Part model, mm, in its own coordinate system. Face numbers are marked on the shaded views. Round coordinates to 2 decimals unless told otherwise and drop trailing zeros. Loops run counter-clockwise (first coordinate to the right, second up) from the corner with the lowest first, then second, coordinate; pieces in that order, holes last. Notation, with made-up numbers: (6.5, -22.75) -> (30.5, -22.75) arc R33 ccw to (30.5, 12.25) -> close; hole circle Ø4 at (1.5, 48). An arc over 180 degrees is marked (long way). Use a Markdown table: item, result. Add a question column.
Item 1: Two-plate mould, pull along Y, no slides. Class the marked faces 1 and 2: pulls with the +Y half, pulls with the -Y half, needs draft (parallel to the pull), parting line crosses it, or undercut.
Item 2: Cut at C-C, the plane z = -21. List the corners of the cut face in (x, y), plus the area to 3 significant figures.
Item 3: Cut at D-D, the plane y = -20. List the corners of the cut face in (x, z).
Item 4: Flat gauge pins, fed straight in: pin 1 (1 mm diameter, centred on x = 1.5, z = -19, fed in from -Y); pin 2 (15 mm diameter, centred on y = 1, z = 5, fed in from -X); pin 3 (1 mm diameter, centred on x = 4, z = 22.5, fed in from +Y); pin 4 (4 mm diameter, centred on y = 0, z = 20, fed in from -X). Where does each tip first touch, or does it go through?
Item 5: Cut at A-A, the plane z = 0. List the corners of the cut face in (x, y).
Item 6: Probe line 1 (Y direction, x = 3.85, z = 0); line 2 (Z direction, x = 4.8, y = -20); line 3 (Y direction, x = 1.4, z = 21). List the from-to ranges inside material, lowest first. Write a range as [from, to].
```python
from build123d import *

# Parameters (mm, degrees)
SKETCH_2_R               = 2.5
CUT_EXTRUDE_1_DEPTH      = 33.3
PATTERN_CIRCULAR_1_COUNT = 4


with BuildPart() as part:
    # Эскиз1 → Повернуть1 (revolve)
    with BuildSketch(Plane.XY, mode=Mode.PRIVATE) as revolve_1_sk:
        Polygon((6, 0), (6, 35), (3, 35), (3, 32), (0, 32), (0, 15), (2, 15), (2, 0), align=None)
    revolve(revolve_1_sk.sketch.rotate(Axis((0, 0, 0), (1, 0, 0)), 90), axis=Axis((0, 0, 0), (1, 0, 0)))

    # Эскиз2 → Вырез-Вытянуть1 (cut)
    with BuildSketch(Plane.ZY):
        with Locations((0, 20)):
            Circle(SKETCH_2_R)
    cut_extrude_1 = extrude(amount=-CUT_EXTRUDE_1_DEPTH, mode=Mode.SUBTRACT)

    # Круговой массив1: Вырез-Вытянуть1 ×4 about axis
    pattern_circular_1_axis = Axis((0, 0, 0), (1, 0, 0))
    for i in range(1, PATTERN_CIRCULAR_1_COUNT):
        add(cut_extrude_1.rotate(pattern_circular_1_axis, i * 360 / PATTERN_CIRCULAR_1_COUNT), mode=Mode.SUBTRACT)


solid = part.part
```
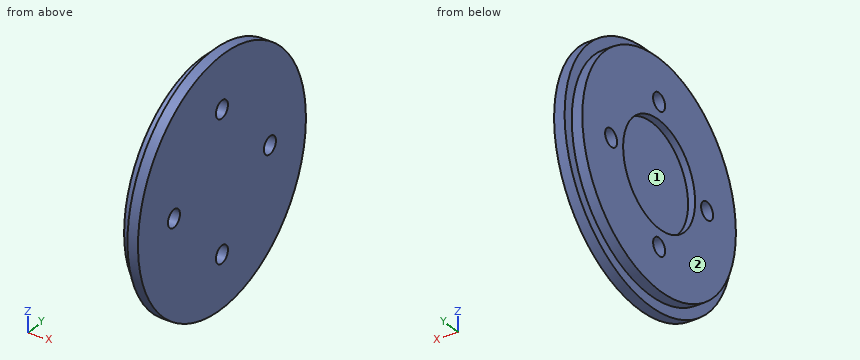
A:
| question | item | result |
|---|---|---|
| 1 | face 1 | undercut |
| 1 | face 2 | needs draft |
| 2 | outline | (0, -24.15) -> (3, -24.15) -> (3, -28) -> (6, -28) -> (6, -2.29) -> (0, -2.29) -> close; (0, 2.29) -> (6, 2.29) -> (6, 28) -> (3, 28) -> (3, 24.15) -> (0, 24.15) -> close |
| 2 | area | 285 mm^2 |
| 3 | outline | (0, -24.98) -> (3, -24.98) -> (3, -28.72) -> (6, -28.72) -> (6, -2.5) -> (0, -2.5) -> close; (0, 2.5) -> (6, 2.5) -> (6, 28.72) -> (3, 28.72) -> (3, 24.98) -> (0, 24.98) -> close |
| 4 | pin 1 | stops at y = -26.11 |
| 4 | pin 2 | stops at x = 2 |
| 4 | pin 3 | stops at y = 27.22 |
| 4 | pin 4 | passes through |
| 5 | outline | (0, -32) -> (3, -32) -> (3, -35) -> (6, -35) -> (6, -22.5) -> (0, -22.5) -> close; (0, -17.5) -> (6, -17.5) -> (6, 17.5) -> (0, 17.5) -> (0, 15) -> (2, 15) -> (2, -15) -> (0, -15) -> close; (0, 22.5) -> (6, 22.5) -> (6, 35) -> (3, 35) -> (3, 32) -> (0, 32) -> close |
| 6 | line 1 | y = [-35, -22.5], [-17.5, 17.5], [22.5, 35] |
| 6 | line 2 | z = [-28.72, -2.5], [2.5, 28.72] |
| 6 | line 3 | y = [-24.15, -2.29], [2.29, 24.15] |
